from build123d import *

# Parameters (mm, degrees)
F0_W     = 63.5
F0_H     = 44.45
F1_DEPTH = 38.1
F2_W     = 19.05
F2_H     = 19.05
F3_DEPTH = 63.501
F4_W     = 31.75
F4_H     = 12.251506
F5_DEPTH = 9.525
F6_W     = 25.4
F6_H     = 12.7
F7_DEPTH = 63.501


with BuildPart() as f1:
    # F0 (on Front) → F1 (new body)
    with BuildSketch(Plane.XZ):
        Rectangle(F0_W, F0_H)
    extrude(amount=F1_DEPTH)

    # F2 (on face) → F3 (cut, through all)
    with BuildSketch(Plane.YZ.offset(31.75)):
        with Locations((-19.05, 12.7)):
            Rectangle(F2_W, F2_H)
    extrude(amount=-F3_DEPTH, mode=Mode.SUBTRACT)

    # F4 (on face) → F5 (cut)
    with BuildSketch(Plane.XZ.offset(38.1)):
        with Locations((0, 16.099247)):
            Rectangle(F4_W, F4_H)
    extrude(amount=-F5_DEPTH, mode=Mode.SUBTRACT)

    # F6 (on face) → F7 (cut, through all)
    with BuildSketch(Plane.YZ.offset(31.75)):
        with Locations((-19.05, -15.875)):
            Rectangle(F6_W, F6_H)
    extrude(amount=-F7_DEPTH, mode=Mode.SUBTRACT)


solid = f1.part
Could you check a few things on this model? Use its own coordinates, in mm. A direction names the side the tool comes from. Give positions to 0.01 mm unless a question says otherwise; leave off trailing zeros. Write each loop counter-clockwise with the first axis right and the second up, starting at its lowest first coordinate (ties: lowest second). Pieces come first, ordered by that corner, then holes. Notation, with made-up numbers: (27, 71.25) -> (37, 71.25) arc R34 cw to (37, 107.25) -> close; hole circle Ø9 at (34, 45.5). An arc over 180 degrees is marked (long way). Answer as CSV lines item,"result". Start each with the question number.
(1) If we section it at A-A, the plane z = 14: Write out the boundary of the cut face in (x, y) (3 decimals).
(2) Please list where these lines run through material, in increasing order: line 1 (Y direction, x = -27, z = 20.5) (3 decimals); line 2 (Y direction, x = 25, z = -15); line 3 (X direction, y = -32, z = 19) (3 decimals).
(3) If we section it at B-B, the plane z = -14: Write out the boundary of the cut face in (x, y).
(4) If we mould it in two halves opening along X, with no side actions, what happens to faces 1 (the face through (-15.875, -33, 16)), 2 (the face through (0, -33, 9.973)), 3 (the face through (0, -35, -22.225)), 4 (the face through (-31.75, -19, 0))? For each: +X half, -X half, draft (parallel to the pull), parting line (faces both ways), or undercut.
(5) Which directions (+Z, -Z, +X, -X, +Y, -Y) give clear straight access to the entire face, cutting with the end or side of a thin tool? Please do faces 5 (the face through (-24, -33, 22.225)), 6 (the face through (15.875, -33, 16)), 7 (the face through (0, -19, -9.525)), 8 (the face through (0, -28.575, 8)).
(6) I'm going to push flat-ended pins straight in: pin 1 Ø8 at (y, z) = (-24, 13.5) entering from -X (3 decimals); pin 2 Ø7.5 at (x, y) = (-9, -22.5) entering from -Z (3 decimals); pin 3 Ø5 at (x, y) = (6, -32) entering from +Z. Where does each tip first touch, or does it pass through?
Answer list:
1,outline,"(-31.75, -38.1) -> (-15.875, -38.1) -> (-15.875, -28.575) -> (-31.75, -28.575) -> close; (-31.75, -9.525) -> (31.75, -9.525) -> (31.75, 0) -> (-31.75, 0) -> close; (15.875, -38.1) -> (31.75, -38.1) -> (31.75, -28.575) -> (15.875, -28.575) -> close"
2,line 1,"-38.1 to -28.575, -9.525 to 0"
2,line 2,"-38.1 to -31.75, -6.35 to 0"
2,line 3,"-31.75 to -15.875, 15.875 to 31.75"
3,outline,"(-31.75, -38.1) -> (31.75, -38.1) -> (31.75, -31.75) -> (-31.75, -31.75) -> close; (-31.75, -6.35) -> (31.75, -6.35) -> (31.75, 0) -> (-31.75, 0) -> close"
4,face 1,"undercut"
4,face 2,"undercut"
4,face 3,"draft"
4,face 4,"-X half"
5,face 5,"+Z, +X, -X, +Y, -Y"
5,face 6,"+Z, -Y"
5,face 7,"-Z, +X, -X"
5,face 8,"+Z, +X, -X"
6,pin 1,"through"
6,pin 2,"z = -9.525"
6,pin 3,"z = 9.97"
